Model file for the job. Use its own axes, mm. Face numbers are marked on the shaded views. A direction names the side the tool comes from. Coordinates: 2 decimals unless noted, no trailing zeros. Loops run counter-clockwise (first coordinate to the right, second up) from the corner with the lowest first, then second, coordinate; pieces in that order, holes last.
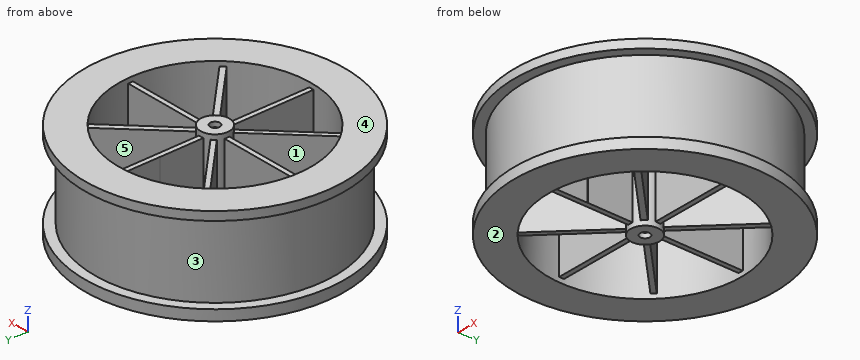
from build123d import *

# Parameters (mm, degrees)
BOX006_W               = 35
BOX006_H               = 1
BOX006_DEPTH           = 18
BOX005_W               = 20
BOX005_H               = 1
BOX005_DEPTH           = 18
BOX004_W               = 45
BOX004_H               = 1
BOX004_DEPTH           = 18
BOX003_W               = 20
BOX003_H               = 1
BOX003_DEPTH           = 18
BOX003_PLACEMENT_ANGLE = 45
BOX002_W               = 35
BOX002_H               = 1
BOX002_DEPTH           = 18
BOX001_W               = 45
BOX001_H               = 1
BOX001_DEPTH           = 18
BOX001_PLACEMENT_ANGLE = 45
BOX_W                  = 20
BOX_H                  = 1
BOX_DEPTH              = 18
BOX_PLACEMENT_ANGLE    = 45
TUBE003_R              = 3
TUBE003_R_2            = 1
TUBE003_DEPTH          = 20
BOX007_W               = 45
BOX007_H               = 1
BOX007_DEPTH           = 18
BOX007_PLACEMENT_ANGLE = 45
TUBE002_R              = 20
TUBE002_R_2            = 2
TUBE002_DEPTH          = 25
TUBE001_R              = 40
TUBE001_R_2            = 25
TUBE001_DEPTH          = 16
TUBE_R                 = 27
TUBE_R_2               = 15
TUBE_DEPTH             = 20


with BuildPart() as cubo006:
    # Box006 → Box006 (new body)
    with BuildSketch(Plane(origin=(-0.6, 12, 1), x_dir=(0, -1, 0), z_dir=(0, 0, 1))):
        with Locations((17.5, 0.5)):
            Rectangle(BOX006_W, BOX006_H)
    extrude(amount=BOX006_DEPTH)


with BuildPart() as cubo005:
    # Box005 → Box005 (new body)
    with BuildSketch(Plane(origin=(1.8, -0.4, 1), x_dir=(1, 0, 0), z_dir=(0, 0, 1))):
        with Locations((10, 0.5)):
            Rectangle(BOX005_W, BOX005_H)
    extrude(amount=BOX005_DEPTH)


with BuildPart() as cubo004:
    # Box004 → Box004 (new body)
    with BuildSketch(Plane(origin=(-22.4, -0.4, 1), x_dir=(1, 0, 0), z_dir=(0, 0, 1))):
        with Locations((22.5, 0.5)):
            Rectangle(BOX004_W, BOX004_H)
    extrude(amount=BOX004_DEPTH)


with BuildPart() as cubo003:
    # Box003 → Box003 (new body)
    with BuildSketch(Plane.XY):
        with Locations((10, 0.5)):
            Rectangle(BOX003_W, BOX003_H)
    extrude(amount=BOX003_DEPTH)


with BuildPart() as cubo003_1:
    # Box003 placement: moved
    add(cubo003.part.moved(Location((2.23, 1.34, 1))).rotate(Axis((2.23, 1.34, 1), (0, 0, 1)), BOX003_PLACEMENT_ANGLE))


with BuildPart() as cubo002:
    # Box002 → Box002 (new body)
    with BuildSketch(Plane(origin=(0.42, -12.28, 1), x_dir=(0, 1, 0), z_dir=(0, 0, 1))):
        with Locations((17.5, 0.5)):
            Rectangle(BOX002_W, BOX002_H)
    extrude(amount=BOX002_DEPTH)


with BuildPart() as cubo001:
    # Box001 → Box001 (new body)
    with BuildSketch(Plane.XY):
        with Locations((22.5, 0.5)):
            Rectangle(BOX001_W, BOX001_H)
    extrude(amount=BOX001_DEPTH)


with BuildPart() as cubo001_1:
    # Box001 placement: moved
    add(cubo001.part.moved(Location((-16.81, -17.43, 1))).rotate(Axis((-16.81, -17.43, 1), (0, 0, 1)), BOX001_PLACEMENT_ANGLE))


with BuildPart() as cubo:
    # Box → Box (new body)
    with BuildSketch(Plane.XY):
        with Locations((10, 0.5)):
            Rectangle(BOX_W, BOX_H)
    extrude(amount=BOX_DEPTH)


with BuildPart() as cubo_1:
    # Box placement: moved
    add(cubo.part.moved(Location((0.75, -1.25, 1))).rotate(Axis((0.75, -1.25, 1), (0, 0, -1)), BOX_PLACEMENT_ANGLE))


with BuildPart() as tube003:
    # Tube003 → Tube003 (new body)
    with BuildSketch(Plane.XY):
        Circle(TUBE003_R)
        Circle(TUBE003_R_2, mode=Mode.SUBTRACT)
    extrude(amount=TUBE003_DEPTH)


with BuildPart() as fusion:
    # Box007 → Box007 (new body)
    with BuildSketch(Plane.XY):
        with Locations((22.5, 0.5)):
            Rectangle(BOX007_W, BOX007_H)
    extrude(amount=BOX007_DEPTH)


with BuildPart() as fusion_1:
    # Box007 placement: moved
    add(fusion.part.moved(Location((-16.706753, 16.006753, 1))).rotate(Axis((-16.706753, 16.006753, 1), (0, 0, -1)), BOX007_PLACEMENT_ANGLE))

    # Fusion: union Cubo006, Cubo005, Cubo004, Cubo003, Cubo002, Cubo001, Cubo, Tube003
    add(cubo006.part)
    add(cubo005.part)
    add(cubo004.part)
    add(cubo003_1.part)
    add(cubo002.part)
    add(cubo001_1.part)
    add(cubo_1.part)
    add(tube003.part)


with BuildPart() as tube002:
    # Tube002 → Tube002 (new body)
    with BuildSketch(Plane.XY.offset(-2.6)):
        Circle(TUBE002_R)
        Circle(TUBE002_R_2, mode=Mode.SUBTRACT)
    extrude(amount=TUBE002_DEPTH)


with BuildPart() as tube001:
    # Tube001 → Tube001 (new body)
    with BuildSketch(Plane.XY.offset(2.2)):
        Circle(TUBE001_R)
        Circle(TUBE001_R_2, mode=Mode.SUBTRACT)
    extrude(amount=TUBE001_DEPTH)


with BuildPart() as fusion001:
    # Tube → Tube (new body)
    with BuildSketch(Plane.XY):
        Circle(TUBE_R)
        Circle(TUBE_R_2, mode=Mode.SUBTRACT)
    extrude(amount=TUBE_DEPTH)

    # Cut: cut Tube001
    add(tube001.part, mode=Mode.SUBTRACT)

    # Cut001: cut Tube002
    add(tube002.part, mode=Mode.SUBTRACT)

    # Fusion001: union Fusion
    add(fusion_1.part)


solid = fusion001.part
Q1. Drill centre lines: line 1 (Y direction, x = 0, z = 19.7); line 2 (X direction, y = -6, z = 17.5). Where is each one in solid material? Low to high.
Answers:
line 1: y = -27 to -20, -3 to -1, 1 to 3, 20 to 27
line 2: x = -24.27 to -19.08, -6.79 to -5.38, -0.6 to 0.42, 5.3 to 6.91, 19.08 to 24.27
Q2. Slice it at D-D (z = 17.25). Count the separate pieces of the cut face and the enclosed holes in it, and give its area (3 significant figures).
Answers:
separate pieces: 1
enclosed holes: 8
area: 877 mm2
Q3. Slice it at C-C (x = -13). List the corners of the cut face in (y, z).
Answers:
outline: (-23.66, 0) - (-15.2, 0) - (-15.2, 20) - (-23.66, 20) - (-23.66, 18.2) - (-21.35, 18.2) - (-21.35, 2.2) - (-23.66, 2.2) - close; (-13.62, 1) - (-12.21, 1) - (-12.21, 19) - (-13.62, 19) - close; (-0.4, 1) - (0.6, 1) - (0.6, 19) - (-0.4, 19) - close; (12.3, 1) - (13.71, 1) - (13.71, 19) - (12.3, 19) - close; (15.2, 0) - (23.66, 0) - (23.66, 2.2) - (21.35, 2.2) - (21.35, 18.2) - (23.66, 18.2) - (23.66, 20) - (15.2, 20) - close
Q4. Which spindle directions (+Z, -Z, +X, -X, +Y, -Y) get a long thin tool onto all of the face, cutting with end or side? Do the marked faces 1 and 2. Say none if no direction does.
Answers:
face 1: +Z, -Z
face 2: -Z, +X, -X, +Y, -Y
Q5. Slice it at B-B (y = -8.5). List the corners of the cut face in (x, z).
Answers:
outline: (-25.63, 0) - (-18.1, 0) - (-18.1, 20) - (-25.63, 20) - (-25.63, 18.2) - (-23.51, 18.2) - (-23.51, 2.2) - (-25.63, 2.2) - close; (-9.29, 1) - (-7.88, 1) - (-7.88, 19) - (-9.29, 19) - close; (-0.6, 1) - (0.42, 1) - (0.42, 19) - (-0.6, 19) - close; (7.8, 1) - (9.41, 1) - (9.41, 19) - (7.8, 19) - close; (18.1, 0) - (25.63, 0) - (25.63, 2.2) - (23.51, 2.2) - (23.51, 18.2) - (25.63, 18.2) - (25.63, 20) - (18.1, 20) - close
Q6. Mould opens along Y. For the marked faces 3, 4 and 5 say: +Y half, -Y half, draft (parallel to the pull), parting line (faces both ways), or undercut.
Answers:
face 3: parting line
face 4: draft
face 5: undercut
Q7. Slice it at A-A (x = 16). List the corners of the cut face in (y, z).
Answers:
outline: (-21.75, 0) - (-12, 0) - (-12, 20) - (-21.75, 20) - (-21.75, 18.2) - (-19.21, 18.2) - (-19.21, 2.2) - (-21.75, 2.2) - close; (-0.4, 1) - (0.6, 1) - (0.6, 19) - (-0.4, 19) - close; (12, 0) - (21.75, 0) - (21.75, 2.2) - (19.21, 2.2) - (19.21, 18.2) - (21.75, 18.2) - (21.75, 20) - (12, 20) - close
Q8. Flat gauge pins, fed straight in: P1, Ø5, axis at x = -20, y = 1.5, coming from the -Z side; P2, Ø2, axis at x = 6, y = 8.5, coming from the +Z side; P3, Ø4, axis at x = 9, z = 4.5, coming from the +Y side; P4, Ø6.5, axis at x = -7, y = -6, coming from the +Z side. Where does each tip first touch, or does it go through?
Answers:
P1: stops at z = 0
P2: passes through
P3: stops at y = 24
P4: stops at z = 19
